Build history of the part. All positions in model axes, mm. Face numbers are marked on the shaded views. A direction names the side the tool comes from. Round coordinates to 2 decimals unless told otherwise and drop trailing zeros. Loops run counter-clockwise (first coordinate to the right, second up) from the corner with the lowest first, then second, coordinate; pieces in that order, holes last. Notation, with made-up numbers: M -36.75,0 L -3.75,0 A14 ccw -3.75,16 Z; hole C 86.5,-20 d6. An arc over 180 degrees is marked long. One line per item, written item: value.
```python
from build123d import *

# Parameters (mm, degrees)
SKETCH_W     = 290
SKETCH_H     = 290
PAD_DEPTH    = 67
THICKNESS_T  = 1
SKETCH001_W  = 50
SKETCH001_H  = 290
PAD001_DEPTH = 37


with BuildPart() as part:
    # Sketch → Pad (new body)
    with BuildSketch(Plane.XY):
        Rectangle(SKETCH_W, SKETCH_H)
    extrude(amount=PAD_DEPTH)

    # Thickness
    thickness_openings = [part.faces().sort_by_distance(p)[0] for p in [
        (0, 0, 67),
    ]]
    offset(amount=THICKNESS_T, openings=thickness_openings)

    # Sketch001 (on Face5 of Thickness) → Pad001 (join)
    with BuildSketch(Plane(origin=(120, 0, 0), x_dir=(1, 0, 0), z_dir=(0, 0, 1))):
        Rectangle(SKETCH001_W, SKETCH001_H)
    pad001 = extrude(amount=PAD001_DEPTH)

    # Mirrored: Pad001 across YZ
    add(pad001.mirror(Plane.YZ))


solid = part.part
```
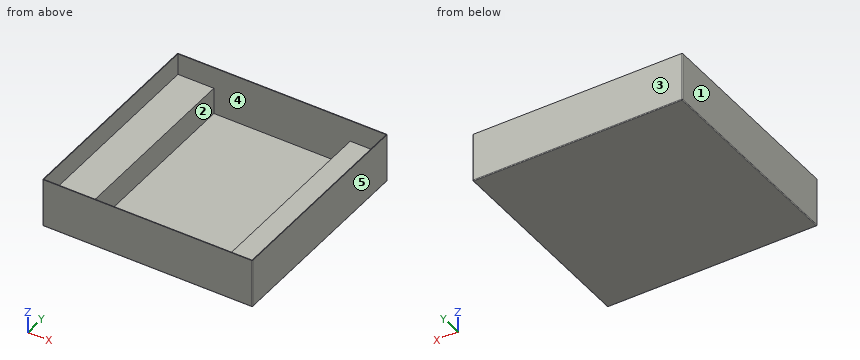
Item 1: Which spindle directions (+Z, -Z, +X, -X, +Y, -Y) get a long thin tool onto all of the face, cutting with end or side? Do the marked faces 4 and 5. Say none if no direction does.
Check values:
face 4: +Z
face 5: +Z, -Z, +X, +Y, -Y
Item 2: Slice it at A-A, the plane z = 61. Give the cut face in (x, y), and give its area (3 significant figures).
Check values:
outline: M -146,-145 A1 ccw -145,-146 L 145,-146 A1 ccw 146,-145 L 146,145 A1 ccw 145,146 L -145,146 A1 ccw -146,145 Z; hole M -145,-145 L 145,-145 L 145,145 L -145,145 Z
area: 1,160 mm2
Item 3: Pull direction Y, two halves, no side cores. Call the marked faces 1, 2 and 3: pulls with the +Y half, pulls with the -Y half, needs draft (parallel to the pull), parting line crosses it, or undercut.
Check values:
face 1: needs draft
face 2: undercut
face 3: pulls with the +Y half
Item 4: Wall check: line 1 along X through (y, z) = (-39, 10); line 2 along Y through (x, z) = (-75.5, 31.5). Give the ranges that are in metal, low to high.
Check values:
line 1: x = -146 to -95, 95 to 146
line 2: y = -146 to -145, 145 to 146
Item 5: Drop flat-ended pins along their axis: P1, Ø2, axis at x = -92, y = -71, coming from the +Z side; P2, Ø15, axis at x = 122, y = -16, coming from the +Z side. Give the stop position or say it passes through.
Check values:
P1: stops at z = 0
P2: stops at z = 37
Item 6: Slice it at C-C, the plane y = 87. Give the cut face in (x, z), and give its area (3 significant figures).
Check values:
outline: M -146,0 A1 ccw -145,-1 L 145,-1 A1 ccw 146,0 L 146,67 L 145,67 L 145,37 L 95,37 L 95,0 L -95,0 L -95,37 L -145,37 L -145,67 L -146,67 Z
area: 4,130 mm2
Item 7: Slice it at D-D, the plane z = 26. Give the cut face in (x, y).
Check values:
outline: M -146,-145 A1 ccw -145,-146 L 145,-146 A1 ccw 146,-145 L 146,145 A1 ccw 145,146 L -145,146 A1 ccw -146,145 Z; hole M -95,-145 L 95,-145 L 95,145 L -95,145 Z
Item 8: Slice it at B-B, the plane x = 5. Give the cut face in (y, z).
Check values:
outline: M -146,0 A1 ccw -145,-1 L 145,-1 A1 ccw 146,0 L 146,67 L 145,67 L 145,0 L -145,0 L -145,67 L -146,67 Z
